Verification items for the finished model (mm, model axes). Coordinates: 2 decimals unless noted, no trailing zeros. Write each loop counter-clockwise with the first axis right and the second up, starting at its lowest first coordinate (ties: lowest second). Pieces come first, ordered by that corner, then holes. Notation, with made-up numbers: (16, 72) - (52, 72) arc R11 ccw to (52, 90) - close; hole circle Ø9 at (-32.5, 42). An arc over 180 degrees is marked (long way). Use one line per item in the form item = value. Start each with the question number.
(1) Material ranges on line 1 (Y direction, x = -139, z = 12.5), recorded low to high. Write a range as [from, to].
(2) Sectioned sample at B-B (y = -234.5). Count the separate pieces of the cut face and the enclosed holes in it, and give its area (3 significant figures).
(3) Gauge pin test, flat ends, axial feed: pin 1 Ø7 at (x, y) = (625, 316.5) entering from -Z; pin 2 Ø8 at (x, z) = (-261.5, 13.5) entering from -Y; pin 3 Ø10 at (x, z) = (37, 25.5) entering from +Y. Record the tip position at first contact, or that the pin passes through.
(4) Sectioned sample at A-A (x = 423.5). Record the cut outline in (y, z), and give its area (3 significant figures).
from build123d import *

# Parameters (mm, degrees)
F0_W     = 40
F0_H     = 0.1
F0_H_2   = 27
F0_W_2   = 900
F0_W_3   = 183
F0_H_3   = 606
F1_DEPTH = 40
F2_T     = -2
F3_DEPTH = 390
F4_R     = 4
F5_DEPTH = 25
F4_R_2   = 6
F6_DEPTH = 40


with BuildPart() as f1:
    # F0 (on Top) → F1 (new body)
    with BuildSketch(Plane.XY):
        with Locations((470, 330.05)):
            Rectangle(F0_W, F0_H)
        with Locations((-470, 330.05)):
            Rectangle(F0_W, F0_H)
        with Locations((470, 316.5)):
            Rectangle(F0_W, F0_H_2)
        with Locations((0, 316.5)):
            Rectangle(F0_W_2, F0_H_2)
        with Locations((-470, 316.5)):
            Rectangle(F0_W, F0_H_2)
        Polygon((450, -330), (700, -330), (700, 330), (490, 330), (490, 303), (450, 303), (450, 47), (-450, 47), (-450, 303), (-490, 303), (-490, 330), (-700, 330), (-700, -330), (-450, -330), (-450, 20), (450, 20), align=None)
        with Locations((-581.5, 0)):
            Rectangle(F0_W_3, F0_H_3, mode=Mode.SUBTRACT)
        with Locations((581.5, 0)):
            Rectangle(F0_W_3, F0_H_3, mode=Mode.SUBTRACT)
    extrude(amount=F1_DEPTH)

    # F2
    f2_openings = [f1.faces().sort_by_distance(p)[0] for p in [
        (-470, 330.1, 20),
        (470, 330.1, 20),
    ]]
    offset(amount=F2_T, openings=f2_openings, kind=Kind.INTERSECTION)

    # F3 (add): faces of the model
    f3_faces = [f1.faces().sort_by_distance(p)[0] for p in [
        (489.4343145751, 330.1, 20),
        (-450.5656854249, 330.1, 20),
    ]]
    extrude(f3_faces, amount=-F3_DEPTH)

    # F4 (on face) → F5 (cut)
    with BuildSketch(Plane(origin=(0, 0, 0), x_dir=(1, 0, 0), z_dir=(0, 0, -1))):
        with Locations((-675, -316.5)):
            Circle(F4_R)
        with Locations((-625, -316.5)):
            Circle(F4_R)
        with Locations((675, -316.5)):
            Circle(F4_R)
        with Locations((625, -316.5)):
            Circle(F4_R)
        with Locations((-675, 316.5)):
            Circle(F4_R)
        with Locations((-625, 316.5)):
            Circle(F4_R)
        with Locations((675, 316.5)):
            Circle(F4_R)
        with Locations((625, 316.5)):
            Circle(F4_R)
    extrude(amount=-F5_DEPTH, mode=Mode.SUBTRACT)

    # F4 (on face) → F6 (join)
    with BuildSketch(Plane(origin=(0, 0, 0), x_dir=(1, 0, 0), z_dir=(0, 0, -1))):
        with Locations((-675, -316.5)):
            Circle(F4_R_2)
        with Locations((-675, -316.5)):
            Circle(F4_R, mode=Mode.SUBTRACT)
        with Locations((-625, -316.5)):
            Circle(F4_R_2)
        with Locations((-625, -316.5)):
            Circle(F4_R, mode=Mode.SUBTRACT)
        with Locations((-675, 316.5)):
            Circle(F4_R_2)
        with Locations((-675, 316.5)):
            Circle(F4_R, mode=Mode.SUBTRACT)
        with Locations((-625, 316.5)):
            Circle(F4_R_2)
        with Locations((-625, 316.5)):
            Circle(F4_R, mode=Mode.SUBTRACT)
        with Locations((675, 316.5)):
            Circle(F4_R_2)
        with Locations((675, 316.5)):
            Circle(F4_R, mode=Mode.SUBTRACT)
        with Locations((625, 316.5)):
            Circle(F4_R_2)
        with Locations((625, 316.5)):
            Circle(F4_R, mode=Mode.SUBTRACT)
        with Locations((675, -316.5)):
            Circle(F4_R_2)
        with Locations((675, -316.5)):
            Circle(F4_R, mode=Mode.SUBTRACT)
        with Locations((625, -316.5)):
            Circle(F4_R_2)
        with Locations((625, -316.5)):
            Circle(F4_R, mode=Mode.SUBTRACT)
    extrude(amount=-F6_DEPTH)


solid = f1.part
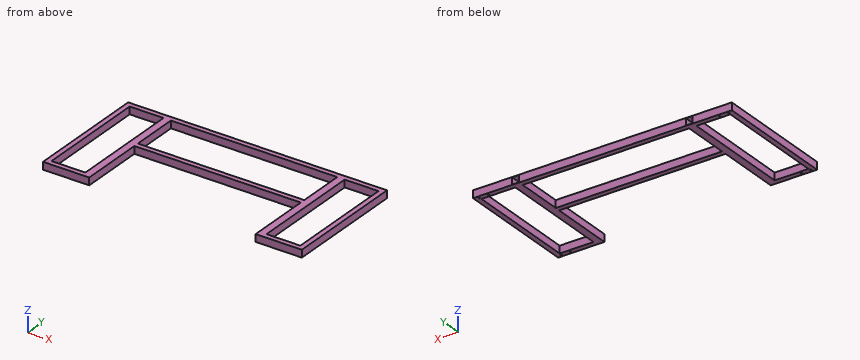
Answers below:
q1.line_1 = [20, 22], [45, 47], [303, 305], [328, 330]
q2.separate_pieces = 4
q2.enclosed_holes = 4
q2.area = 1,110 mm2
q3.pin_1 = 38
q3.pin_2 = 20
q3.pin_3 = 330
q4.outline = (20, 0) - (47, 0) - (47, 40) - (20, 40) - close; (303, 0) - (330, 0) - (330, 40) - (303, 40) - close; hole (22, 2) - (45, 2) - (45, 38) - (22, 38) - close; hole (305, 2) - (328, 2) - (328, 38) - (305, 38) - close
q4.area = 504 mm2
